Work out the finished part from the listing and answer in its coordinate system (mm). A direction names the side the tool comes from. Round coordinates to 2 decimals unless told otherwise and drop trailing zeros. Use a Markdown table: item, result. Add a question column.
Item 1: Find the intervals of material crossed by L1, parallel to X at y = -73.5, z = 20.75, in increasing order. Write a range as [from, to].
Item 2: A tool of negligible diameter and unlimited length cuts with its end or side. For faces 4 (the flat face through (1, -144.259, 12)), 5 (the cylindrical face through (-17.641, -73.087, 18.916)), from which of +Z, -Z, +X, -X, +Y, -Y can it reach the whole face along a straight path? Write none if from no direction.
Item 3: For a pull along Y with two mould halves and no side action, classify faces 1 (the flat face through (1, -45.944, 12)), 2 (the flat face through (1, -94, 0)), 3 (the conical face through (-53.51, -83.24, 11.76)) as +Y half, -Y half, draft (parallel to the pull), parting line (faces both ways), or undercut.
from build123d import *

# Parameters (mm, degrees)
F0_W     = 113.3287157863
F0_H     = 98.3149297535
F1_DEPTH = 25
F4_D     = 5
F4_DEPTH = 12
F4_TIP   = 1.5021515476


with BuildPart() as f1:
    # F0 (on Top) → F1 (new body)
    with BuildSketch(Plane.XY):
        with Locations((-44.8288666084, -95.1015558094)):
            Rectangle(F0_W, F0_H)
    extrude(amount=F1_DEPTH)

    # F2: F1 across plane


with BuildPart() as f1_1:
    add(f1.part)
    add(f1.part.mirror(Plane.YZ))

    # F4
    with Locations(Plane.XY.offset(25)):
        with Locations((-53.4110553563, -82.8184708953), (-17.9668162018, -75.5653455853)):
            Hole(F4_D / 2, depth=F4_DEPTH)
            with Locations((0, 0, -(F4_DEPTH + F4_TIP / 2))):  # 118° drill point
                Cone(0, F4_D / 2, F4_TIP, mode=Mode.SUBTRACT)


solid = f1_1.part
Reported:
| question | item | result |
|---|---|---|
| 1 | L1 | [-101.49, -19.38], [-16.56, 101.49] |
| 2 | face 4 | +Z, -Z, +X, -X, -Y |
| 2 | face 5 | +Z |
| 3 | face 1 | +Y half |
| 3 | face 2 | draft |
| 3 | face 3 | undercut |
